Check sheet for the modelled part. Datum: model origin and axes. Units: mm. A direction names the side the tool comes from. Round coordinates to 2 decimals unless told otherwise and drop trailing zeros. Order: outer loops, then holes, each group sorted by start corner. A loop starts at its lowest first (then second) coordinate and runs counter-clockwise, first axis right, second up. Notation, with made-up numbers: (10, 84) -> (50, 84) arc R28 ccw to (50, 113) -> close; hole circle Ø9 at (-11.75, 57). An arc over 180 degrees is marked (long way). Answer in a Markdown table with one row per item.
```python
from build123d import *

# Parameters (mm, degrees)
SKETCH1_R           = 37.084
BOSS_EXTRUDE1_DEPTH = 12.7
SKETCH2_R           = 35.814
BOSS_EXTRUDE2_DEPTH = 3.048
SKETCH3_R           = 40.386
BOSS_EXTRUDE3_DEPTH = 48.26
FILLET1_R           = 2.54
FILLET2_R           = 5.08
FILLET3_R           = 2.032


with BuildPart() as part:
    # Sketch1 → Boss-Extrude1 (new body)
    with BuildSketch(Plane.XY):
        Circle(SKETCH1_R)
    extrude(amount=BOSS_EXTRUDE1_DEPTH)

    # Sketch2 → Boss-Extrude2 (add)
    with BuildSketch(Plane(origin=(0, 0, 0), x_dir=(-1, 0, 0), z_dir=(0, 0, -1))):
        with Locations(Location((0, 0, 0), (0, 0, 180))):
            Circle(SKETCH2_R)
    extrude(amount=BOSS_EXTRUDE2_DEPTH)

    # Sketch3 → Boss-Extrude3 (add)
    with BuildSketch(Plane(origin=(0, 0, -3.048), x_dir=(-1, 0, 0), z_dir=(0, 0, -1))):
        with Locations(Location((0, 0, 0), (0, 0, 180))):
            Circle(SKETCH3_R)
    extrude(amount=BOSS_EXTRUDE3_DEPTH)

    # Fillet1
    fillet1_edges = [part.edges().sort_by_distance(p)[0] for p in [
        (-40.386, 0, -3.048),
    ]]
    fillet(fillet1_edges, radius=FILLET1_R)

    # Fillet2
    fillet2_edges = [part.edges().sort_by_distance(p)[0] for p in [
        (-40.386, 0, -51.308),
    ]]
    fillet(fillet2_edges, radius=FILLET2_R)

    # Fillet3
    # the kernel refuses this fillet: 2.032 mm, written as the material it takes off along each edge
    with BuildSketch(Plane(origin=(0, 0, 0), x_dir=(1, 0, 0), z_dir=(0, -1, 0))) as fillet3_piece_1:
        with BuildLine():
            CenterArc((35.052, 1.883714416), FILLET3_R, 292.024312837, 67.975687163)
            Line((37.084, 1.883714416), (37.12464, 1.883714416))
            Line((37.12464, 1.883714416), (37.12464, 0))
            Line((37.12464, 0), (37.084, -0.04064))
            ThreePointArc((37.084, -0.04064), (36.449, -0.04064), (35.82924, -0.037674288))
            Line((35.82924, -0.037674288), (35.814, 0))
        make_face()
    revolve(axis=Axis((0, 0, 0), (0, 0, 1)), mode=Mode.SUBTRACT)
    with BuildSketch(Plane(origin=(0, 0, 12.7), x_dir=(1, 0, 0), z_dir=(0, -1, 0))) as fillet3_piece_2:
        with BuildLine():
            CenterArc((37.084 - FILLET3_R, -FILLET3_R), FILLET3_R, 0, 90)
            Line((37.084 - FILLET3_R, 0), (37.084 - FILLET3_R, FILLET3_R * 0.02))
            Line((37.084 - FILLET3_R, FILLET3_R * 0.02), (37.084 + FILLET3_R * 0.02, FILLET3_R * 0.02))
            Line((37.084 + FILLET3_R * 0.02, FILLET3_R * 0.02), (37.084 + FILLET3_R * 0.02, -FILLET3_R))
            Line((37.084 + FILLET3_R * 0.02, -FILLET3_R), (37.084, -FILLET3_R))
        make_face()
    revolve(axis=Axis((0, 0, 12.7), (0, 0, 1)), mode=Mode.SUBTRACT)


solid = part.part
```
(1) Scan lines: probe 1 along Y at (x, z) = (-16, -7); probe 2 along Y at (x, z) = (-23.5, -8.5). Record each from-to range of solid material in increasing order. Write a range as from..to.
Solutions:
| item | result |
|---|---|
| probe 1 | -37.08..37.08 |
| probe 2 | -32.84..32.84 |
(2) Draft check along Z on faces 1 (the cylindrical face through (-7.764, 34.962, -1.503)), 2 (the flat face through (0, 0, -51.308)), 3 (the cylindrical face through (-27.3, 25.1, 6.2)). Enter one of: pulls with the +Z half, pulls with the -Z half, needs draft (parallel to the pull), parting line crosses it, or undercut.
Solutions:
| item | result |
|---|---|
| face 1 | undercut |
| face 2 | pulls with the -Z half |
| face 3 | needs draft |
(3) Depth check by flat-ended pin: pin 1 Ø2 at (x, z) = (32, -11) entering from +Y; pin 2 Ø10 at (x, z) = (3, -22) entering from +Y; pin 3 Ø10 at (x, z) = (-21.5, -13) entering from -Y. Enter the tip coordinate at first touch or a pass-through.
Solutions:
| item | result |
|---|---|
| pin 1 | y = 25.88 |
| pin 2 | y = 40.39 |
| pin 3 | y = -36.86 |
(4) Tool access check on faces 4 (the flat face through (0, 0, 12.7)), 5 (the flat face through (-23, 28, -3.048)). Record the directions out of +Z, -Z, +X, -X, +Y, -Y that give a thin tool (end or side, any length) a straight path to the whole face; none if there is none.
Solutions:
| item | result |
|---|---|
| face 4 | +Z, +X, -X, +Y, -Y |
| face 5 | none |
(5) Section check C-C on z = -17. Record the boundary of the cut face in (x, y).
Solutions:
| item | result |
|---|---|
| outline | circle Ø80.77 at (0, 0) |
(6) Section check A-A on y = 0. Record the boundary of the cut face in (x, z), plus the area to 3 significant figures.
Solutions:
| item | result |
|---|---|
| outline | (-40.39, -46.23) arc R5.08 ccw to (-35.31, -51.31) -> (35.31, -51.31) arc R5.08 ccw to (40.39, -46.23) -> (40.39, -5.59) arc R2.54 ccw to (37.85, -3.05) -> (35.81, -3.05) -> (35.81, 0) arc R2.03 ccw to (37.08, 1.88) -> (37.08, 10.67) arc R2.03 ccw to (35.05, 12.7) -> (-35.05, 12.7) arc R2.03 ccw to (-37.08, 10.67) -> (-37.08, 1.88) arc R2.03 ccw to (-35.81, 0) -> (-35.81, -3.05) -> (-37.85, -3.05) arc R2.54 ccw to (-40.39, -5.59) -> close |
| area | 5,040 mm^2 |
